Source: CAD feature listing. Evaluate the final solid. Frame: model axes, mm. A direction names the side the tool comes from. Give positions to 0.01 mm unless a question says otherwise; leave off trailing zeros. Loops run counter-clockwise (first coordinate to the right, second up) from the corner with the lowest first, then second, coordinate; pieces in that order, holes last. Notation, with made-up numbers: M 24.25,49 L 77.25,49 A12 cw 77.25,57 Z; hole C 2.25,-5 d6. An arc over 180 degrees is marked long. Put each result on its own line as item: value.
from build123d import *

# Parameters (mm, degrees)
SKETCH1_W                    = 40
SKETCH1_H                    = 38
SKETCH1_R                    = 7
SKETCH1_R_2                  = 1.5
BASE_FLANGE1_DEPTH           = 2
EDGE_FLANGE1_STRIP_W         = 10
EDGE_FLANGE1_STRIP_H         = 2
EDGE_FLANGE1_STRIP_CUT_DEPTH = 40
EDGE_FLANGE1_DEPTH           = 40
FILLET1_R                    = 10
FILLET2_R                    = 3
SKETCH10_R                   = 1.5
CUT_EXTRUDE1_DEPTH           = 49.023431781


# Sheet-metal steps are written as plain solids
with BuildPart() as part:
    # Sketch1 → Base-Flange1 (new body)
    with BuildSketch(Plane(origin=(0, 0, 0), x_dir=(1, 0, 0), z_dir=(0, 1, 0))):
        Rectangle(SKETCH1_W, SKETCH1_H)
        with Locations(Location((0, -1, 0), (0, 0, 270))):
            Circle(SKETCH1_R, mode=Mode.SUBTRACT)
        with Locations(Location((0, -10.5, 0), (0, 0, 270))):
            Circle(SKETCH1_R_2, mode=Mode.SUBTRACT)
    extrude(amount=-BASE_FLANGE1_DEPTH)

    # Edge-Flange1 strip (across the edge) → Edge-Flange1 strip cut (cut)
    with BuildSketch(Plane(origin=(-20, 0, 19), x_dir=(0, 0, -1), z_dir=(1, 0, 0))):
        with Locations((-4, -1)):
            Rectangle(EDGE_FLANGE1_STRIP_W, EDGE_FLANGE1_STRIP_H)
    extrude(amount=EDGE_FLANGE1_STRIP_CUT_DEPTH, mode=Mode.SUBTRACT)

    # Edge-Flange1 section (across the edge) → Edge-Flange1 (add)
    with BuildSketch(Plane(origin=(-20, 0, 19), x_dir=(0, 0, -1), z_dir=(1, 0, 0))):
        with BuildLine():
            Line((-2, 1), (-2, 21.5))
            Line((-2, 21.5), (0, 21.5))
            Line((0, 21.5), (0, 1))
            ThreePointArc((0, 1), (0.292893219, 0.292893219), (1, 0))
            Line((1, 0), (1, -2))
            ThreePointArc((1, -2), (-1.121320344, -1.121320344), (-2, 1))
        make_face()
    extrude(amount=EDGE_FLANGE1_DEPTH)

    # Fillet1
    fillet1_edges = [part.edges().sort_by_distance(p)[0] for p in [
        (-20, -1, -19),
        (20, -1, -19),
    ]]
    fillet(fillet1_edges, radius=FILLET1_R)

    # Fillet2
    fillet2_edges = [part.edges().sort_by_distance(p)[0] for p in [
        (-20, 21.5, 20),
        (20, 21.5, 20),
    ]]
    fillet(fillet2_edges, radius=FILLET2_R)

    # Sketch10 → Cut-Extrude1 (cut, through all)
    with BuildSketch(Plane(origin=(0, 0, 19), x_dir=(-1, 0, 0), z_dir=(0, 0, -1))):
        with Locations((-14.5, 16.5)):
            Circle(SKETCH10_R)
        with Locations((-14.5, 10.5)):
            Circle(SKETCH10_R)
        with Locations((-14.5, 4.5)):
            Circle(SKETCH10_R)
        with Locations(Location((14.5, 4.5, 0), (0, 0, 180))):
            Circle(SKETCH10_R)
        with Locations(Location((14.5, 10.5, 0), (0, 0, 180))):
            Circle(SKETCH10_R)
        with Locations(Location((14.5, 16.5, 0), (0, 0, 180))):
            Circle(SKETCH10_R)
    extrude(amount=-CUT_EXTRUDE1_DEPTH, mode=Mode.SUBTRACT)


solid = part.part
1. Draft query along X for faces 1 (the cylindrical face through (0, -1, 9)), 2 (the cylindrical face through (16, 4.57, 19.99)), 3 (the cylindrical face through (19.1, 20.64, 19.99)), 4 (the flat face through (-5, -2, -5)). Return one class per face: pulls with the +X half, pulls with the -X half, needs draft (parallel to the pull), parting line crosses it, or undercut.
Found:
face 1: undercut
face 2: undercut
face 3: pulls with the +X half
face 4: needs draft
2. Material intervals for line 1 (X direction, y = -1.1, z = 1); line 2 (Y direction, x = 14.5, z = 19.95); line 3 (Z direction, x = -14, y = 19.25), sorted ascending. Write a range as from..to.
Found:
line 1: -20..-7, 7..20
line 2: -1.28..3, 6..9, 12..15, 18..21.5
line 3: 19..21
3. Section query A-A (y = 4.5). Output: boundary loops of the cut face in (x, z), plus the area to 3 significant figures.
Found:
outline: M -20,19 L -16,19 L -16,21 L -20,21 Z; M -13,19 L 13,19 L 13,21 L -13,21 Z; M 16,19 L 20,19 L 20,21 L 16,21 Z
area: 68.0 mm^2
4. Section query C-C (x = 0). Output: boundary loops of the cut face in (y, z), plus the area to 3 significant figures.
Found:
outline: M -2,-19 L 0,-19 L 0,-6 L -2,-6 Z; M -2,8 L 0,8 L 0,9 L -2,9 Z; M -2,12 L 0,12 L 0,18 A1 cw 1,19 L 21.5,19 L 21.5,21 L 1,21 A3 ccw -2,18 Z
area: 87.3 mm^2
5. Access query for faces 5 (the cylindrical face through (-19.14, 20.6, 19.99)), 6 (the flat face through (0, 11, 19)). Directions: +Z, -Z, +X, -X, +Y, -Y. A direction counts if a zero-diameter tool reaches every point of the face in a straight line with its end or side. Return the directions, or none.
Found:
face 5: +Z, -Z, -X, +Y
face 6: -Z, +X, -X, +Y
6. Section query B-B (z = 10.5). Output: boundary loops of the cut face in (x, y).
Found:
outline: M -20,-2 L -1.5,-2 L -1.5,0 L -20,0 Z; M 1.5,-2 L 20,-2 L 20,0 L 1.5,0 Z
7. Contact query for flat-ended pins moving along their axis: P1, Ø10, axis at x = -5.5, z = -13, coming from the +Y side; P2, Ø10, axis at x = -2, y = 11.5, coming from the -Z side; P3, Ø1.8, axis at x = -14.5, y = 16.5, coming from the +Z side. Output: stop coordinate, or through.
Found:
P1: y = 0
P2: z = 19
P3: through
8. Section query D-D (x = -14.5). Output: boundary loops of the cut face in (y, z).
Found:
outline: M -2,-17.93 L 0,-17.93 L 0,18 A1 cw 1,19 L 3,19 L 3,21 L 1,21 A3 ccw -2,18 Z; M 6,19 L 9,19 L 9,21 L 6,21 Z; M 12,19 L 15,19 L 15,21 L 12,21 Z; M 18,19 L 21.5,19 L 21.5,21 L 18,21 Z
